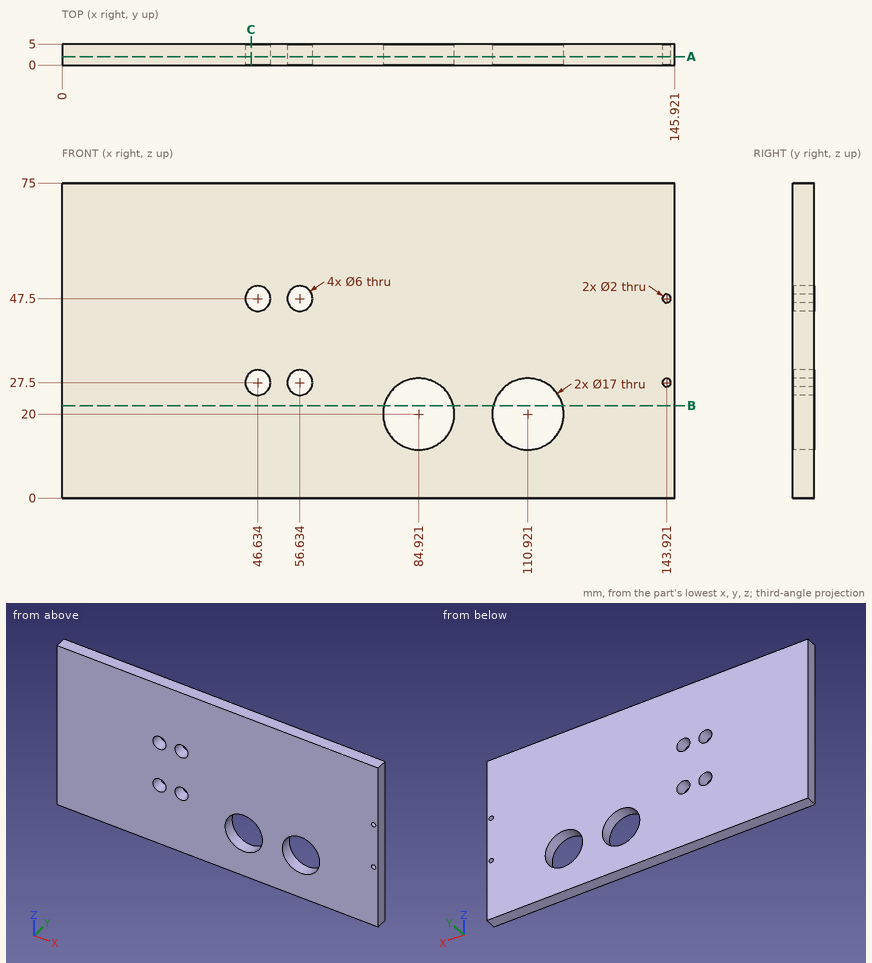
Job drawing, mm, ordinate dimensions from the low corner. One solid piece. Coordinates: 2 decimals unless noted, no trailing zeros. Loops run counter-clockwise (first coordinate to the right, second up) from the corner with the lowest first, then second, coordinate; pieces in that order, holes last. Notation, with made-up numbers: (74, 24) - (132, 24) arc R33 ccw to (132, 63) - close; hole circle Ø4 at (30, -21). An arc over 180 degrees is marked (long way). Answer as a JSON object with one key per item and string values. Group by question number.
(1) Probe line 1 along X through (y, z) = (2.95, 47) (1 decimal); line 2 along X through (y, z) = (4.1, 25.5); line 3 along X through (y, z) = (1.55, 15.5). List the from-to ranges inside material, lowest first.
(2) Cut at C-C (x = 45). Give the cut face in (y, z).
(3) Cut at B-B (z = 22). Give the cut face in (x, y).
(4) Cut at A-A (y = 2). State how many separate pieces and enclosed holes the cut face has, then the cut area to 3 significant figures.
(5) Flat gauge pin, fed straight in: pin 1 (12 mm diameter, centred on x = 101, z = 59, fed in from -Y). Where does the tip first touch, or does it go through?
Geometry says:
{
 "1": {"line 1": "x = 0 to 43.7, 49.6 to 53.7, 59.6 to 143.1, 144.8 to 145.9", "line 2": "x = 0 to 44.4, 48.87 to 54.4, 58.87 to 78.44, 91.4 to 104.44, 117.4 to 145.92", "line 3": "x = 0 to 77.71, 92.13 to 103.71, 118.13 to 145.92"},
 "2": {"outline": "(0, 0) - (5, 0) - (5, 24.98) - (0, 24.98) - close; (0, 30.02) - (5, 30.02) - (5, 44.98) - (0, 44.98) - close; (0, 50.02) - (5, 50.02) - (5, 75) - (0, 75) - close"},
 "3": {"outline": "(0, 0) - (76.66, 0) - (76.66, 5) - (0, 5) - close; (93.18, 0) - (102.66, 0) - (102.66, 5) - (93.18, 5) - close; (119.18, 0) - (145.92, 0) - (145.92, 5) - (119.18, 5) - close"},
 "4": {"separate pieces": "1", "enclosed holes": "8", "area": "10,400 mm^2"},
 "5": {"pin 1": "stops at y = 0"}
}
